Source: three-view drawing plus pictorial views. Frame: mm from the lowest corner of the part. A direction names the side the tool comes from. Give positions to 0.01 mm unless a question says otherwise; leave off trailing zeros. Loops run counter-clockwise (first coordinate to the right, second up) from the corner with the lowest first, then second, coordinate; pieces in that order, holes last.
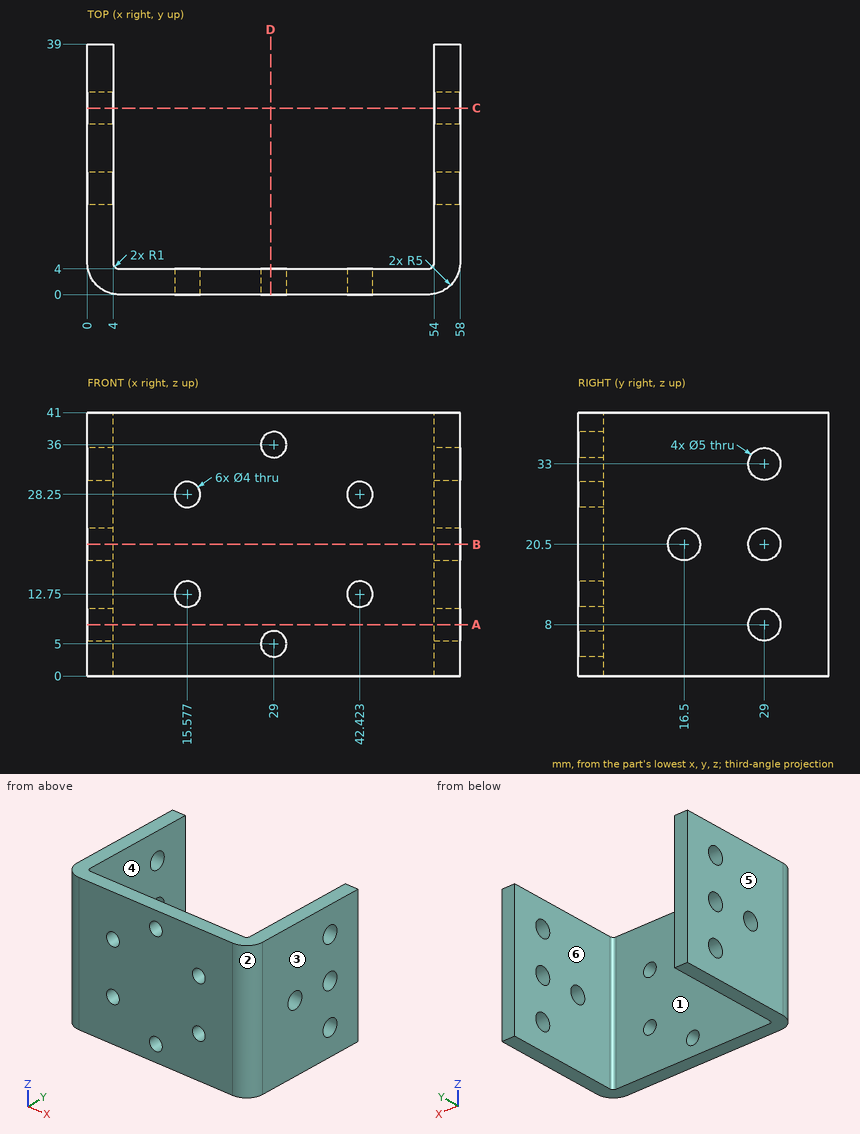
Q1. Section query A-A, the plane z = 8. Return loops of the section in (x, y).
Q2. Section query C-C, the plane y = 29. State how many separate pieces and enclosed holes the cut face has, and give its area (3 significant figures).
Q3. Mould query, pull axis X, two halves, no side actions, for the marked faces 3, 4, 5 and 6. Classes: +X half, -X half, draft (parallel to the pull), parting line (faces both ways), or undercut.
Q4. Reachability of the marked faces 1 and 2 from +Z, -Z, +X, -X, +Y, -Y: full face, straight path, thin tool, end or side. Return the list, or none.
Q5. Material intervals for probe 1 along X at (y, z) = (32, 25); probe 2 along X at (y, z) = (3, 28); probe 3 along Y at (x, z) = (55.1, 20.5), sorted ascending.
Q6. Pin query (flat end, axial travel): pin 1 Ø4.5 at (y, z) = (16.5, 20.5) entering from +X; pin 2 Ø2 at (x, z) = (20, 8.5) entering from +Y; pin 3 Ø1.5 at (y, z) = (21.5, 36) entering from -X. Return the tip coordinate at first contact, or that it passes through.
Q7. Section query B-B, the plane z = 20.5. Return loops of the section in (x, y).
Q8. Section query D-D, the plane x = 28.5. Return loops of the section in (y, z), and give its area (3 significant figures).
Resolved:
1. outline: (0, 5) arc R5 ccw to (5, 0) - (53, 0) arc R5 ccw to (58, 5) - (58, 26.5) - (54, 26.5) - (54, 5) arc R1 cw to (53, 4) - (5, 4) arc R1 cw to (4, 5) - (4, 26.5) - (0, 26.5) - close; (0, 31.5) - (4, 31.5) - (4, 39) - (0, 39) - close; (54, 31.5) - (58, 31.5) - (58, 39) - (54, 39) - close
2. separate pieces: 8
2. enclosed holes: 0
2. area: 208 mm2
3. face 3: +X half
3. face 4: undercut
3. face 5: -X half
3. face 6: undercut
4. face 1: +Z, -Z, +Y
4. face 2: +Z, -Z, +X, -Y
5. probe 1: x = 0 to 4, 54 to 58
5. probe 2: x = 0.42 to 13.59, 17.56 to 40.44, 44.41 to 57.58
5. probe 3: y = 0.46 to 14, 19 to 26.5, 31.5 to 39
6. pin 1: passes through
6. pin 2: stops at y = 4
6. pin 3: stops at x = 0
7. outline: (0, 5) arc R5 ccw to (5, 0) - (53, 0) arc R5 ccw to (58, 5) - (58, 14) - (54, 14) - (54, 5) arc R1 cw to (53, 4) - (5, 4) arc R1 cw to (4, 5) - (4, 14) - (0, 14) - close; (0, 19) - (4, 19) - (4, 26.5) - (0, 26.5) - close; (0, 31.5) - (4, 31.5) - (4, 39) - (0, 39) - close; (54, 19) - (58, 19) - (58, 26.5) - (54, 26.5) - close; (54, 31.5) - (58, 31.5) - (58, 39) - (54, 39) - close
8. outline: (0, 0) - (4, 0) - (4, 3.06) - (0, 3.06) - close; (0, 6.94) - (4, 6.94) - (4, 34.06) - (0, 34.06) - close; (0, 37.94) - (4, 37.94) - (4, 41) - (0, 41) - close
8. area: 133 mm2
